Read the model definition and answer for the solid it produces. Units are mm, in the model's axes. Face numbers are marked on the shaded views. A direction names the side the tool comes from. Coordinates: 2 decimals unless noted, no trailing zeros. Loops run counter-clockwise (first coordinate to the right, second up) from the corner with the lowest first, then second, coordinate; pieces in that order, holes last. Notation, with made-up numbers: (78, -12.5) - (87, -12.5) arc R10 cw to (87, -1.5) - close; hole circle Ø5 at (66, 71). An arc over 180 degrees is marked (long way). Use one line per item in the form item = value. Start each with the question number.
1) A cutting plane is placed at B-B (y = 57). Give the vertices of the cut face in (x, z), and give its area (3 significant figures).
2) A cutting plane is placed at D-D (y = 270). Give the vertices of the cut face in (x, z), and give its area (3 significant figures).
3) Consider line 1 (Y direction, x = 126.5, z = 31); line 2 (X direction, y = -39.5, z = 203.5); line 3 (Z direction, x = -177.5, y = 164.5). Determine where each line is inside the solid, lowest interval first.
4) A cutting plane is placed at A-A (z = 161.5). Give the vertices of the cut face in (x, y), and give its area (3 significant figures).
5) Which of the six approach directions +Z, -Z, +X, -X, +Y, -Y give full straight-line access (tool end or side, diameter ignored) to the marked faces 1 and 2?
6) A cutting plane is placed at C-C (z = 66.5). Give the vertices of the cut face in (x, y).
7) The mould has two halves that part along X. Classify the marked faces 3, 4 and 5: released by +X, released by -X, zero draft, split by the parting line, or undercut.
8) Each of these flat-tipped pins is pushed along its axis until it touches: P1, Ø0.6, axis at x = 119.5, y = -83, coming from the -Z side; P2, Ø0.6, axis at x = 128.5, y = -82.5, coming from the +Z side; P3, Ø1.9, axis at x = 184, z = 144, coming from the -Y side. Where does it stop, or does it pass through?
from build123d import *

# Parameters (mm, degrees)
F0_W          = 381
F0_H          = 381
F1_DEPTH      = 6.35
F2_W          = 393.7
F2_H          = 393.7
F2_W_2        = 381
F2_H_2        = 381
F3_DEPTH      = 304.8
F3_DEPTH_BACK = 6.35
F4_W          = 91.44
F4_H          = 172.72
F5_DEPTH      = 25.4
F6_W          = 165.1
F6_H          = 50.8
F7_DEPTH      = 25.4
F8_W          = 31.75
F8_H          = 12.7
F9_DEPTH      = 1.27
F8_W_2        = 35.56
F8_H_2        = 16.51
F10_DEPTH     = 1.905


with BuildPart() as f1:
    # F0 (on Top) → F1 (new body)
    with BuildSketch(Plane.XY):
        with Locations((-9.435589, 114.986119)):
            Rectangle(F0_W, F0_H)
    extrude(amount=F1_DEPTH)

    # F2 (on face) → F3 (join, two sides)
    with BuildSketch(Plane.XY.offset(6.35)) as f3_sk:
        with Locations((-9.435589, 114.986119)):
            Rectangle(F2_W, F2_H)
        with Locations((-9.435589, 114.986119)):
            Rectangle(F2_W_2, F2_H_2, mode=Mode.SUBTRACT)
    extrude(amount=F3_DEPTH)
    extrude(f3_sk.sketch, amount=-F3_DEPTH_BACK)

    # F4 (on face) → F5 (cut)
    with BuildSketch(Plane.XZ.offset(81.863881)):
        with Locations((51.556636, 92.71)):
            Rectangle(F4_W, F4_H)
    extrude(amount=-F5_DEPTH, mode=Mode.SUBTRACT)

    # F6 (on face) → F7 (cut)
    with BuildSketch(Plane.YZ.offset(187.414411)):
        Polygon((32.436119, 155.575), (32.436119, 152.4), (197.536119, 152.4), (197.536119, 203.2), (32.436119, 203.2), align=None)
        with Locations((114.986119, 127)):
            Rectangle(F6_W, F6_H)
    extrude(amount=-F7_DEPTH, mode=Mode.SUBTRACT)

    # F8 (on face) → F9 (join)
    with BuildSketch(Plane.XZ.offset(81.863881)):
        with Locations((120.726646, 114.625568)):
            Rectangle(F8_W, F8_H)
    extrude(amount=F9_DEPTH)

    # F8 (on face) → F10 (join)
    with BuildSketch(Plane.XZ.offset(81.863881)):
        with Locations((120.726646, 114.625568)):
            Rectangle(F8_W_2, F8_H_2)
        with Locations((120.726646, 114.625568)):
            Rectangle(F8_W, F8_H, mode=Mode.SUBTRACT)
    extrude(amount=F10_DEPTH)


solid = f1.part
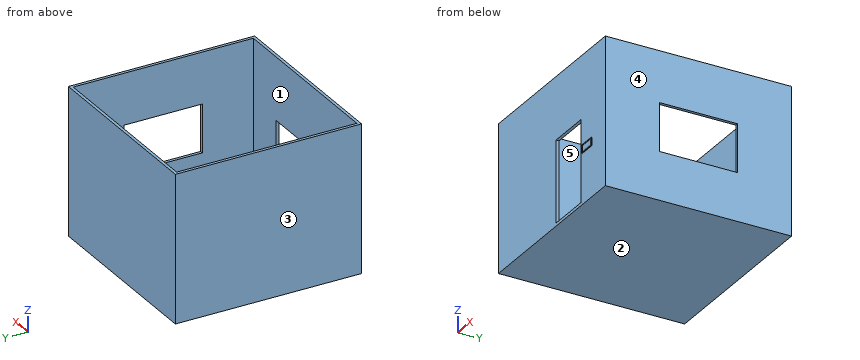
Found:
q1.outline = (-206.29, 0) - (187.41, 0) - (187.41, 101.6) - (181.06, 101.6) - (181.06, 6.35) - (-199.94, 6.35) - (-199.94, 311.15) - (-206.29, 311.15) - close; (181.06, 203.2) - (187.41, 203.2) - (187.41, 311.15) - (181.06, 311.15) - close
q1.area = 5,730 mm^2
q2.outline = (-206.29, 0) - (187.41, 0) - (187.41, 311.15) - (181.06, 311.15) - (181.06, 6.35) - (-199.94, 6.35) - (-199.94, 311.15) - (-206.29, 311.15) - close
q2.area = 6,370 mm^2
q3.line_1 = -81.86 to -75.51, 305.49 to 311.84
q3.line_2 = -206.29 to -199.94, 181.06 to 187.41
q3.line_3 = 0 to 6.35
q4.outline = (-206.29, -81.86) - (5.84, -81.86) - (5.84, -75.51) - (-199.94, -75.51) - (-199.94, 305.49) - (181.06, 305.49) - (181.06, 197.54) - (187.41, 197.54) - (187.41, 311.84) - (-206.29, 311.84) - close; (97.28, -81.86) - (187.41, -81.86) - (187.41, 32.44) - (181.06, 32.44) - (181.06, -75.51) - (97.28, -75.51) - close
q4.area = 8,210 mm^2
q5.face_1 = +Z
q5.face_2 = -Z, +X, -X, +Y, -Y
q6.outline = (-206.29, -81.86) - (5.84, -81.86) - (5.84, -75.51) - (-199.94, -75.51) - (-199.94, 305.49) - (181.06, 305.49) - (181.06, -75.51) - (97.28, -75.51) - (97.28, -81.86) - (187.41, -81.86) - (187.41, 311.84) - (-206.29, 311.84) - close
q7.face_3 = released by -X
q7.face_4 = released by +X
q7.face_5 = undercut
q8.P1 = 106.37
q8.P2 = 122.88
q8.P3 = -81.86
